The listing builds one solid part. Answer for the finished solid, in the listing's coordinates (mm). A direction names the side the tool comes from. Coordinates: 2 decimals unless noted, no trailing zeros. Loops run counter-clockwise (first coordinate to the right, second up) from the corner with the lowest first, then second, coordinate; pieces in that order, holes last. Notation, with made-up numbers: M 54.5,-25.75 L 85.5,-25.75 A22 ccw 85.5,5.25 Z; hole C -15,-12 d2. An arc over 180 degrees is marked long. Return JSON: item names as keys, results as strings. Group by question number.
1. Given P1, Ø1.5, axis at y = 972.5, z = 33.5, coming from the +X side; P2, Ø3, axis at x = 429, z = 51, coming from the +Y side; P3, Ø11, axis at x = 902.5, z = 7, coming from the +Y side, each flat-ended and moving along its own axis, determine where each tip first touches the part or whether it passes through.
2. The mould has two halves that part along X. Classify faces 4 (the face through (1175, 44, 9)), 5 (the face through (75, 1035, 49)), 6 (the face through (114, 2100, 9)): pulls with the +X half, pulls with the -X half, needs draft (parallel to the pull), parting line crosses it, or undercut.
3. Section B-B (x = 147.5) is taken. Write down the section's boundary in (y, z), then the cut area to 3 significant figures.
4. Section A-A (z = 41.5) is taken. Write down the section's boundary in (x, y).
5. Straight lines are drawn through the part: L1, parallel to Y at x = 320.5, z = 52.5; L2, parallel to X at y = 285, z = 9.5; L3, parallel to X at y = 1283, z = 48.5. For each, find the intervals that lie inside material, in ascending order. Write a range as from..to.
6. Section C-C (y = 880.5) is taken. Write down the section's boundary in (x, z).
7. Which of the six approach directions +Z, -Z, +X, -X, +Y, -Y give full straight-line access (tool end or side, diameter ignored) to faces 1 (the face through (633, 0, 49)), 2 (the face through (183, 750, 10)), 3 (the face through (83.22, 119.44, 29.37))?
```python
from build123d import *

# Parameters (mm, degrees)
PAD_DEPTH       = 100
SKETCH001_W     = 1090
SKETCH001_H     = 2090
POCKET_DEPTH    = 90
POCKET001_DEPTH = 50


with BuildPart() as part:
    # Sketch → Pad (new body)
    with BuildSketch(Plane.XY):
        Polygon((75, 0), (75, 2100), (215, 2100), (215, 140), (1175, 140), (1175, 0), align=None)
    extrude(amount=PAD_DEPTH)

    # Sketch001 (on Face8 of Pad) → Pocket (cut)
    with BuildSketch(Plane.XY.offset(100)):
        with Locations((630, 1055)):
            Rectangle(SKETCH001_W, SKETCH001_H)
    extrude(amount=-POCKET_DEPTH, mode=Mode.SUBTRACT)

    # Sketch002 (on Face1 of Pocket) → Pocket001 (cut)
    with BuildSketch(Plane(origin=(75, 0, 0), x_dir=(0, -1, 0), z_dir=(-1, 0, 0))):
        with BuildLine():
            ThreePointArc((-95.588953, 77.406408), (-97.362834, 94.284037), (-114.240456, 92.510097))
            ThreePointArc((-114.240456, 92.510097), (-138.568299, 49.069608), (-147, 0))
            Line((-147, 0), (-123, 0))
            ThreePointArc((-95.588953, 77.406408), (-115.944903, 41.058244), (-123, 0))
        make_face()
    extrude(amount=-POCKET001_DEPTH, mode=Mode.SUBTRACT)


solid = part.part
```
Worked out:
{
 "1": {"P1": "x = 85", "P2": "y = 10", "P3": "y = 140"},
 "2": {"face 4": "pulls with the +X half", "face 5": "pulls with the -X half", "face 6": "needs draft"},
 "3": {"outline": "M 0,0 L 2100,0 L 2100,10 L 10,10 L 10,100 L 0,100 Z", "area": "21,900 mm^2"},
 "4": {"outline": "M 75,0 L 1175,0 L 1175,10 L 85,10 L 85,115.79 L 75,115.79 Z; M 75,141.02 L 85,141.02 L 85,2100 L 75,2100 Z"},
 "5": {"L1": "0..10", "L2": "75..215", "L3": "75..85"},
 "6": {"outline": "M 75,0 L 215,0 L 215,10 L 85,10 L 85,100 L 75,100 Z"},
 "7": {"face 1": "+Z, -Z, +X, -X, -Y", "face 2": "+Z, +X, +Y", "face 3": "-X"}
}
